from build123d import *

# Parameters (mm, degrees)
F0_R     = 18.5
F0_R_2   = 12.5
F1_DEPTH = 7
F2_R     = 14.015719
F2_R_2   = 13.698062
F3_DEPTH = 0.254
F4_R     = 17.024352
F4_R_2   = 16.672097
F5_DEPTH = 0.254
F6_R     = 20
F6_R_2   = 18.5
F7_DEPTH = 1.5


with BuildPart() as f1:
    # F0 (on Top) → F1 (new body)
    with BuildSketch(Plane.XY):
        Circle(F0_R)
        Circle(F0_R_2, mode=Mode.SUBTRACT)
    extrude(amount=F1_DEPTH)

    # F2 (on face) → F3 (cut)
    with BuildSketch(Plane.XY.offset(7)):
        Circle(F2_R)
        Circle(F2_R_2, mode=Mode.SUBTRACT)
    extrude(amount=-F3_DEPTH, mode=Mode.SUBTRACT)

    # F4 (on face) → F5 (cut)
    with BuildSketch(Plane.XY.offset(7)):
        Circle(F4_R)
        Circle(F4_R_2, mode=Mode.SUBTRACT)
    extrude(amount=-F5_DEPTH, mode=Mode.SUBTRACT)

    # F6 (on face) → F7 (join)
    with BuildSketch(Plane.XY.offset(7)):
        Circle(F6_R)
        Circle(F6_R_2, mode=Mode.SUBTRACT)
    extrude(amount=-F7_DEPTH)


solid = f1.part
Input: part model. Units: mm. Frame: model coordinates. A direction names the side the tool comes from. Give positions to 0.01 mm unless a question says otherwise; leave off trailing zeros. Write each loop counter-clockwise with the first axis right and the second up, starting at its lowest first coordinate (ties: lowest second). Pieces come first, ordered by that corner, then holes. Notation, with made-up numbers: M 22,-38.75 L 72,-38.75 A13 cw 72,-24.75 Z; hole C 69,51 d10. An arc over 180 degrees is marked long. Use one line per item in the form item = value.
1. Ray query, L1, parallel to Y at x = 0, z = 6.8; L2, parallel to X at y = 0.5, z = 6; L3, parallel to Y at x = 0, z = 3.5. Return the intervals inside material, ascending.
Outcome:
L1 = -20 to -17.02, -16.67 to -14.02, -13.7 to -12.5, 12.5 to 13.7, 14.02 to 16.67, 17.02 to 20
L2 = -19.99 to -12.49, 12.49 to 19.99
L3 = -18.5 to -12.5, 12.5 to 18.5
2. Reachability of faces 5 (the face through (11.3, -12.5, 6.746)), 6 (the face through (15, 9, 7)) from +Z, -Z, +X, -X, +Y, -Y: full face, straight path, thin tool, end or side. Return the list, or none.
Outcome:
face_5 = +Z
face_6 = +Z, +X, -X, +Y, -Y
3. First-contact query: P1, Ø1, axis at x = -2, z = 1, coming from the -Y side; P2, Ø20, axis at x = 6.5, y = 2.5, coming from the -Z side; P3, Ø1.5, axis at y = 8.5, z = 1, coming from the -X side; P4, Ø3, axis at y = 12, z = 2, coming from the -X side. Flat tips, straight axial feed; report the tip coordinate or a pass-through.
Outcome:
P1 = -18.44
P2 = 0
P3 = -16.8
P4 = -15.23
4. Mould query, pull axis Y, two halves, no side actions, for faces 1 (the face through (11.923, 3.755, 3.451)), 2 (the face through (6, -18, 5.5)), 3 (the face through (-4.01, -18.06, 2.71)), 4 (the face through (6.2, -12.4, 6.746)). Classes: released by +Y, released by -Y, zero draft, split by the parting line, or undercut.
Outcome:
face_1 = undercut
face_2 = zero draft
face_3 = split by the parting line
face_4 = undercut
5. Cut plane A-A on y = 0. Return loops of the section in (x, z).
Outcome:
outline = M -20,5.5 L -18.5,5.5 L -18.5,0 L -12.5,0 L -12.5,7 L -13.7,7 L -13.7,6.75 L -14.02,6.75 L -14.02,7 L -16.67,7 L -16.67,6.75 L -17.02,6.75 L -17.02,7 L -20,7 Z; M 12.5,0 L 18.5,0 L 18.5,5.5 L 20,5.5 L 20,7 L 17.02,7 L 17.02,6.75 L 16.67,6.75 L 16.67,7 L 14.02,7 L 14.02,6.75 L 13.7,6.75 L 13.7,7 L 12.5,7 Z
6. Cut plane C-C on z = 0.5. Return loops of the section in (x, y).
Outcome:
outline = C 0,0 d37; hole C 0,0 d25
